Geometry check sheet. Reference: the model listing, model coordinates, mm. Face numbers are marked on the shaded views. A direction names the side the tool comes from. Round coordinates to 2 decimals unless told otherwise and drop trailing zeros. Loops run counter-clockwise (first coordinate to the right, second up) from the corner with the lowest first, then second, coordinate; pieces in that order, holes last. Notation, with made-up numbers: (71, -5.75) -> (104, -5.75) arc R21 ccw to (104, 5.25) -> close; hole circle Ø4 at (-9.5, 56.5). An arc over 180 degrees is marked (long way). Use one line per item in the form item = value.
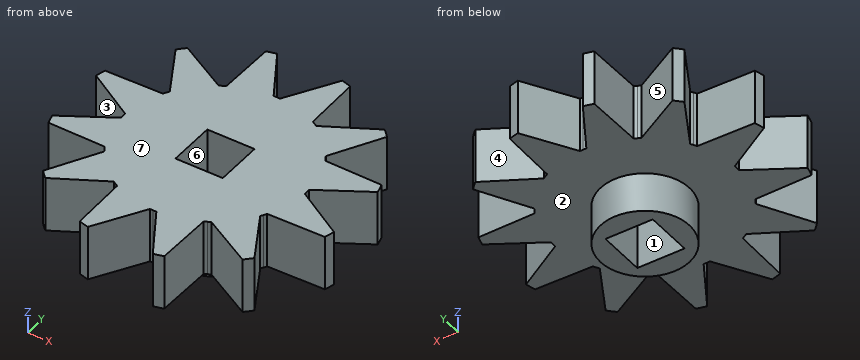
from build123d import *

# Parameters (mm, degrees)
F0_R            = 11
F1_DEPTH        = 4.2
F3_DEPTH        = 4.201
F3_COPIES_COUNT = 12
F5_R            = 3.3858769499
F6_DEPTH        = 3
F7_W            = 3.6
F7_H            = 3.6
F8_DEPTH        = 7.201


# Not quite as in the source:
# - a pattern or mirror of a feature is missing from the dataset's text; its kind, count and spacing are read off the source's solid


with BuildPart() as f1:
    # F0 (on Top) → F1 (new body)
    with BuildSketch(Plane.XY):
        Circle(F0_R)
    extrude(amount=F1_DEPTH)

    # F2 (on face) → F3 (cut, through all)
    with BuildSketch(Plane(origin=(0, 0, 0), x_dir=(1, 0, 0), z_dir=(0, 0, -1))):
        with BuildLine():
            ThreePointArc((-0.2442964769, 6.9957357891), (-0.1221668451, 6.9989338661), (0, 7))
            Line((0, 7), (0, 11))
            ThreePointArc((0, 11), (-1.2452353514, 10.9292904124), (-2.4744615978, 10.7180707126))
            Line((-2.4744615978, 10.7180707126), (-0.2442964769, 6.9957357891))
        make_face()
        with BuildLine():
            Line((0, 11), (0, 7))
            ThreePointArc((0, 7), (0.1221668451, 6.9989338661), (0.2442964769, 6.9957357891))
            Line((0.2442964769, 6.9957357891), (2.4744615978, 10.7180707126))
            ThreePointArc((2.4744615978, 10.7180707126), (1.2452353514, 10.9292904124), (0, 11))
        make_face()
    f3 = extrude(amount=-F3_DEPTH, mode=Mode.SUBTRACT)

    # F3_copies: F3 ×12 about axis
    f3_copies_axis = Axis((0, 0, 0), (0, 0, 1))
    for i in range(1, F3_COPIES_COUNT):
        add(f3.rotate(f3_copies_axis, i * 360 / F3_COPIES_COUNT), mode=Mode.SUBTRACT)

    # F5 (on face) → F6 (join)
    with BuildSketch(Plane(origin=(0, 0, 0), x_dir=(1, 0, 0), z_dir=(0, 0, -1))):
        Circle(F5_R)
    extrude(amount=F6_DEPTH)

    # F7 (on face) → F8 (cut, through all)
    with BuildSketch(Plane(origin=(0, 0, -3), x_dir=(1, 0, 0), z_dir=(0, 0, -1))):
        Rectangle(F7_W, F7_H)
    extrude(amount=-F8_DEPTH, mode=Mode.SUBTRACT)


solid = f1.part
1. Section check B-B (x = 9.5). Record the boundary of the cut face in (y, z).
Return value:
outline = (-3.23, 0) -> (-1.74, 0) -> (-1.74, 4.2) -> (-3.23, 4.2) -> close; (1.74, 0) -> (3.23, 0) -> (3.23, 4.2) -> (1.74, 4.2) -> close
2. Section check C-C (x = -5.25). Record the boundary of the cut face in (y, z), then the cut area to 3 significant figures.
Return value:
outline = (-6.79, 0) -> (6.79, 0) -> (6.79, 4.2) -> (-6.79, 4.2) -> close
area = 57.1 mm2
3. Mould release check, pull along Y, two halves, no side actions. Record for the marked faces 5, 6 and 7: released by +Y, released by -Y, zero draft, split by the parting line, or undercut.
Return value:
face_5 = released by +Y
face_6 = undercut
face_7 = zero draft
4. Section check A-A (z = -1). Record the boundary of the cut face in (x, y), then the cut area to 3 significant figures.
Return value:
outline = circle Ø6.77 at (0, 0); hole (-1.8, -1.8) -> (1.8, -1.8) -> (1.8, 1.8) -> (-1.8, 1.8) -> close
area = 23.1 mm2
5. Tool access check on the marked faces 1, 2, 3 and 4. Record the directions out of +Z, -Z, +X, -X, +Y, -Y that give a thin tool (end or side, any length) a straight path to the whole face; none if there is none.
Return value:
face_1 = +Z, -Z
face_2 = -Z
face_3 = +Z, -Z, -X
face_4 = +Z, -Z, +Y
6. Gauge pin test, flat ends, axial feed: pin 1 (2 mm diameter, centred on x = -3.5, z = 0, fed in from -Y); pin 2 (1 mm diameter, centred on x = -4, z = 0.5, fed in from -Y); pin 3 (4 mm diameter, centred on x = 0, z = 1, fed in from +Y). Record the tip position at first contact, or that the pin passes through.
Return value:
pin_1 = -10.71
pin_2 = -6.38
pin_3 = 9.93
7. Material ranges on line 1 along Y through (x, z) = (6.75, 2); line 2 along X through (y, z) = (-6.25, 2); line 3 along Y through (x, z) = (-3.5, 0.75), recorded low to high.
Return value:
line_1 = -7.63 to -5.17, -3.28 to 3.28, 5.17 to 7.63
line_2 = -7.35 to -4.27, -3.29 to 3.29, 4.27 to 7.35
line_3 = -6.06 to 6.06
